from build123d import *

# Parameters (mm, degrees)
SKETCH1_W           = 20
SKETCH1_H           = 28
BOSS_EXTRUDE1_DEPTH = 5
SKETCH2_R           = 1.5
CUT_EXTRUDE1_DEPTH  = 5
SKETCH3_W           = 16
SKETCH3_H           = 3
CUT_EXTRUDE2_DEPTH  = 20
SKETCH4_W           = 16
SKETCH4_H           = 10
CUT_EXTRUDE3_DEPTH  = 4


with BuildPart() as part:
    # Sketch1 → Boss-Extrude1 (new body)
    with BuildSketch(Plane.XY):
        with Locations((10, 14)):
            Rectangle(SKETCH1_W, SKETCH1_H)
    extrude(amount=BOSS_EXTRUDE1_DEPTH)

    # Sketch2 → Cut-Extrude1 (cut)
    with BuildSketch(Plane.XY.offset(5)):
        with Locations((10, 4)):
            Circle(SKETCH2_R)
    extrude(amount=-CUT_EXTRUDE1_DEPTH, mode=Mode.SUBTRACT)

    # Sketch3 → Cut-Extrude2 (cut)
    with BuildSketch(Plane(origin=(0, 28, 0), x_dir=(1, 0, 0), z_dir=(0, 1, 0))):
        with Locations((10, -2.5)):
            Rectangle(SKETCH3_W, SKETCH3_H)
    extrude(amount=-CUT_EXTRUDE2_DEPTH, mode=Mode.SUBTRACT)

    # Sketch4 → Cut-Extrude3 (cut)
    with BuildSketch(Plane.XY.offset(5)):
        with Locations((10, 13)):
            Rectangle(SKETCH4_W, SKETCH4_H)
    extrude(amount=-CUT_EXTRUDE3_DEPTH, mode=Mode.SUBTRACT)


solid = part.part
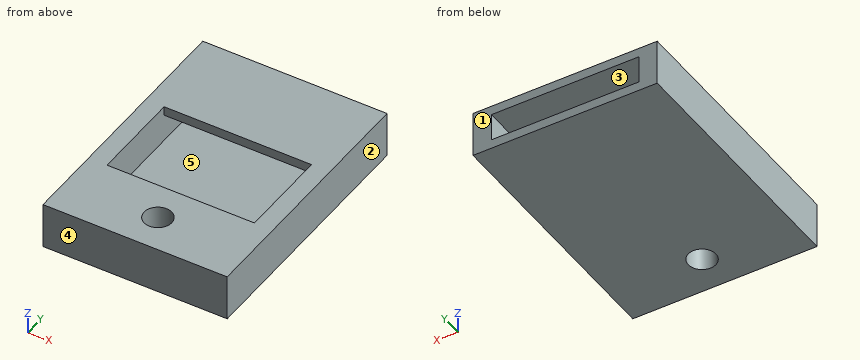
Check sheet for the modelled part. Datum: model origin and axes. Units: mm. Face numbers are marked on the shaded views. A direction names the side the tool comes from. Give positions to 0.01 mm unless a question says otherwise; leave off trailing zeros. Write each loop counter-clockwise with the first axis right and the second up, starting at its lowest first coordinate (ties: lowest second). Pieces come first, ordered by that corner, then holes. Notation, with made-up numbers: (18, 50.25) -> (47, 50.25) arc R20 ccw to (47, 61.25) -> close; hole circle Ø4 at (16.5, 64.25). An arc over 180 degrees is marked (long way). One line per item, written item: value. Start each with the question number.
Item 1: Section check C-C on x = 10. Record the cut outline in (y, z), then the cut area to 3 significant figures.
Item 2: Section check B-B on z = 2.1. Record the cut outline in (x, y), then the cut area to 3 significant figures.
Item 3: Material ranges on probe 1 along X at (y, z) = (24, 1.45); probe 2 along Y at (x, z) = (10, 1.65); probe 3 along Z at (x, y) = (8.25, 23.25), recorded low to high. Write a range as from..to.
Item 4: Tool access check on the marked faces 4 and 5. Record the directions out of +Z, -Z, +X, -X, +Y, -Y that give a thin tool (end or side, any length) a straight path to the whole face; none if there is none.
Item 5: Section check D-D on y = 12. Record the cut outline in (x, z), then the cut area to 3 significant figures.
Item 6: Section check A-A on y = 4. Record the cut outline in (x, z).
Item 7: Draft check along X on the marked faces 1, 2 and 3. Enter one of: +X half, -X half, draft (parallel to the pull), parting line (faces both ways), or undercut.
Results list:
1. outline: (0, 0) -> (2.5, 0) -> (2.5, 5) -> (0, 5) -> close; (5.5, 0) -> (28, 0) -> (28, 1) -> (8, 1) -> (8, 5) -> (5.5, 5) -> close; (18, 4) -> (28, 4) -> (28, 5) -> (18, 5) -> close
1. area: 55.0 mm²
2. outline: (0, 0) -> (20, 0) -> (20, 28) -> (18, 28) -> (18, 8) -> (2, 8) -> (2, 28) -> (0, 28) -> close; hole circle Ø3 at (10, 4)
2. area: 233 mm²
3. probe 1: 0..2, 18..20
3. probe 2: 0..2.5, 5.5..8
3. probe 3: 0..1, 4..5
4. face 4: +Z, -Z, +X, -X, -Y
4. face 5: +Y
5. outline: (0, 0) -> (20, 0) -> (20, 5) -> (18, 5) -> (18, 1) -> (2, 1) -> (2, 5) -> (0, 5) -> close
5. area: 36.0 mm²
6. outline: (0, 0) -> (8.5, 0) -> (8.5, 5) -> (0, 5) -> close; (11.5, 0) -> (20, 0) -> (20, 5) -> (11.5, 5) -> close
7. face 1: draft
7. face 2: +X half
7. face 3: undercut
